from build123d import *

# Parameters (mm, degrees)
F0_R     = 43.18
F1_DEPTH = 508
F4_R     = 25.4
F5_R     = 12.7
F6_DEPTH = 508.001


with BuildPart() as f1:
    # F0 (on Top) → F1 (new body)
    with BuildSketch(Plane.XY):
        Circle(F0_R)
    extrude(amount=F1_DEPTH)

    # F2 (on Front) → F3 (revolve, cut)
    with BuildSketch(Plane.XZ):
        with BuildLine():
            Line((-384.330451, 258.428335), (-98.216951, 75.272329))
            ThreePointArc((-98.216951, 75.272329), (-22.933279, 256.891851), (-93.24689, 440.492717))
            Line((-93.24689, 440.492717), (-384.330451, 258.428335))
        make_face()
    revolve(axis=Axis((0, 0, 0), (0, 0, -1)), mode=Mode.SUBTRACT)

    # F4
    f4_edges = [f1.edges().sort_by_distance(p)[0] for p in [
        (0, -43.18, 158.762324),
        (0, 43.18, 158.762324),
        (-22.908703, 0, 260.503948),
        (0, 43.18, 362.245572),
        (0, -43.18, 362.245572),
    ]]
    fillet(f4_edges, radius=F4_R)

    # F5 (on face) → F6 (cut, through all)
    with BuildSketch(Plane(origin=(0, 0, 0), x_dir=(1, 0, 0), z_dir=(0, 0, -1))):
        Circle(F5_R)
    extrude(amount=-F6_DEPTH, mode=Mode.SUBTRACT)


solid = f1.part
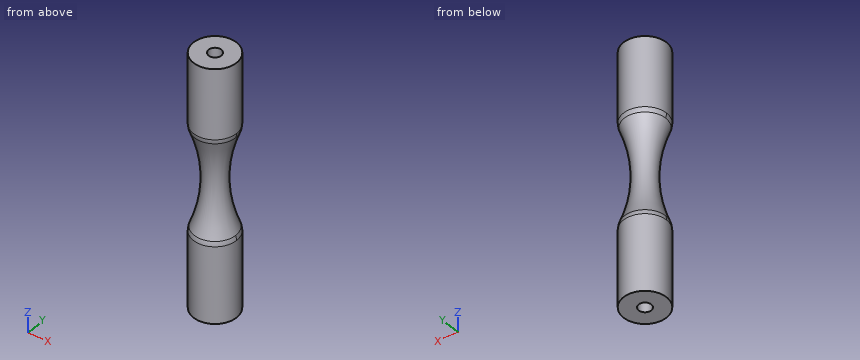
Model file for the job. Use its own axes, mm. Give positions to 0.01 mm unless a question says otherwise; leave off trailing zeros. Loops run counter-clockwise (first coordinate to the right, second up) from the corner with the lowest first, then second, coordinate; pieces in that order, holes last.
Item 1: Drill centre lines: line 1 along Y through (x, z) = (0, 118.5); line 2 along X through (y, z) = (-1, 373); line 3 along X through (y, z) = (0, 291). Where is each one in solid material? Low to high.
Check values:
line 1: y = -43.18 to -12.7, 12.7 to 43.18
line 2: x = -43.17 to -12.66, 12.66 to 43.17
line 3: x = -24.67 to -12.7, 12.7 to 24.67
Item 2: Slice it at A-A (z = 397.5). Write the cut outline in (x, y).
Check values:
outline: circle Ø86.36 at (0, 0); hole circle Ø25.4 at (0, 0)
Item 3: Slice it at B-B (z = 213). Write the cut outline in (x, y).
Check values:
outline: circle Ø54.39 at (0, 0); hole circle Ø25.4 at (0, 0)
Item 4: Drop flat-ended pins along their axis: P1, Ø6, axis at x = -16, y = -18.5, coming from the -Z side; P2, Ø12, axis at x = 32, z = 155, coming from the +Y side; P3, Ø6, axis at x = 16.5, z = 135.5, coming from the +Y side; P4, Ø1, axis at y = -19.5, z = 87, coming from the +X side. Give the stop position or say it passes through.
Check values:
P1: stops at z = 0
P2: stops at y = 34.45
P3: stops at y = 41.02
P4: stops at x = 38.78
